Verification items for this drawing (mm, ordinates from the low corner). Give positions to 0.01 mm unless a question says otherwise; leave off trailing zeros. Write each loop counter-clockwise with the first axis right and the second up, starting at its lowest first coordinate (ties: lowest second). Pieces come first, ordered by that corner, then holes. Notation, with made-up numbers: (43.5, 4) -> (94.5, 4) arc R17 ccw to (94.5, 19) -> close; hole circle Ø1 at (58, 85.25). An arc over 180 degrees is marked (long way). Write item = value, one per line.
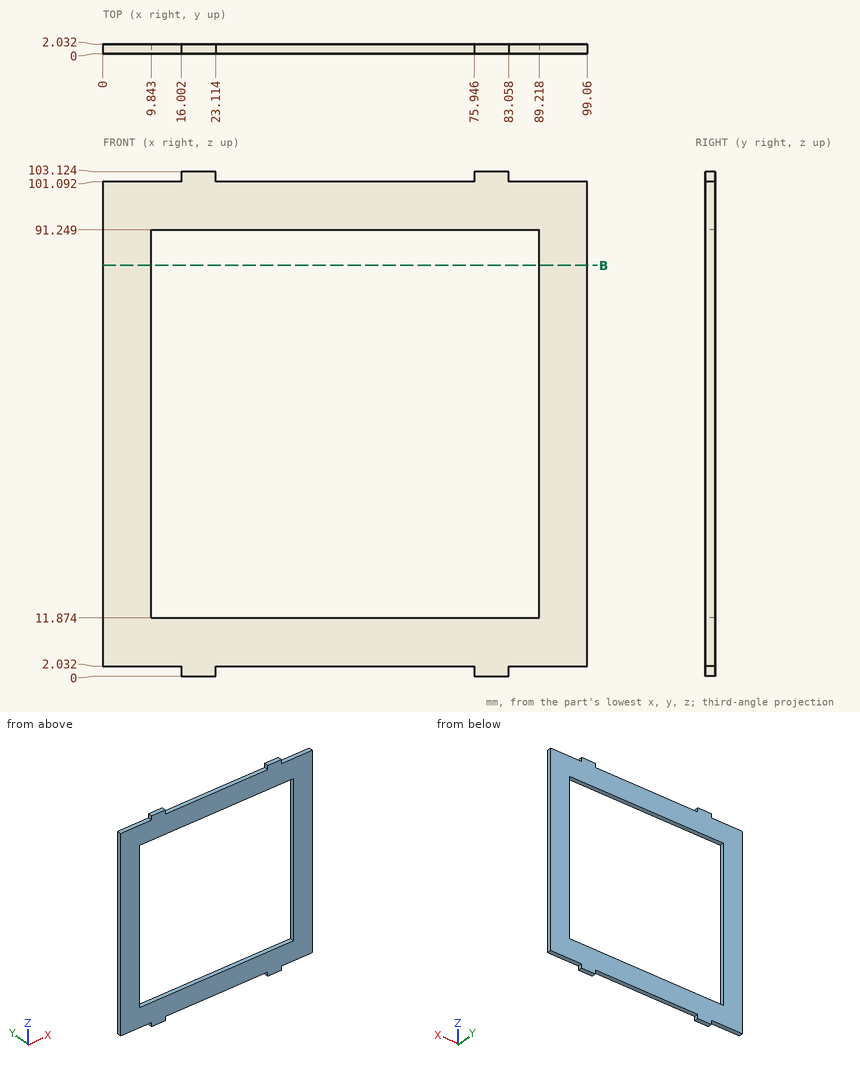
Item 1: Material ranges on line 1 (X direction, y = 0.8, z = 90); line 2 (Z direction, x = 6, y = 0.35), recorded low to high.
Response values:
line_1 = 0 to 9.84, 89.22 to 99.06
line_2 = 2.03 to 101.09
Item 2: Go/stop test with flat-tipped pins: P1, Ø0.6, axis at x = 8.5, y = 1, coming from the -Z side; P2, Ø1, axis at y = 1, z = 1, coming from the +X side; P3, Ø1, axis at x = 5, y = 1.5, coming from the +Z side. Record where each tip stops, or that it passes through.
Response values:
P1 = 2.03
P2 = 83.06
P3 = 101.09
Item 3: Sectioned sample at B-B on z = 84. Record the cut outline in (x, y), then the cut area to 3 significant figures.
Response values:
outline = (0, 0) -> (9.84, 0) -> (9.84, 2.03) -> (0, 2.03) -> close; (89.22, 0) -> (99.06, 0) -> (99.06, 2.03) -> (89.22, 2.03) -> close
area = 40.0 mm^2
